Geometry: see drawing. Coordinates: mm, zero at the bounding-box minimum. Round coordinates to 2 decimals unless told otherwise and drop trailing zeros. Loops run counter-clockwise (first coordinate to the right, second up) from the corner with the lowest first, then second, coordinate; pieces in that order, holes last. Notation, with made-up numbers: (2.5, 28) - (57.5, 28) arc R22 ccw to (57.5, 49) - close; hole circle Ø7 at (-22, 88). An arc over 180 degrees is marked (long way). Return JSON: item names as keys, results as strings. Group by question number.
1. Material intervals for probe 1 along Y at (x, z) = (35, 3.45); probe 2 along Y at (x, z) = (35, 0.8); probe 3 along Z at (x, y) = (34, 43), sorted ascending.
2. First-contact query: pin 1 Ø3.5 at (x, y) = (35, 41.5) entering from +Z; pin 2 Ø3 at (y, z) = (30, 4) entering from +X; pin 3 Ø3 at (y, z) = (9, 1.5) entering from -X (3 decimals). Flat tips, straight axial feed; report the tip coordinate or a pass-through.
3. Section B-B on y = 35. Return loops of the section in (x, z), and give its area (3 significant figures).
4. Section C-C on z = 4.9. Return loops of the section in (x, y), and give its area (3 significant figures).
5. Section A-A on x = 35. Return loops of the section in (y, z).
6. Section D-D on y = 55. Return loops of the section in (x, z), and give its area (3 significant figures).
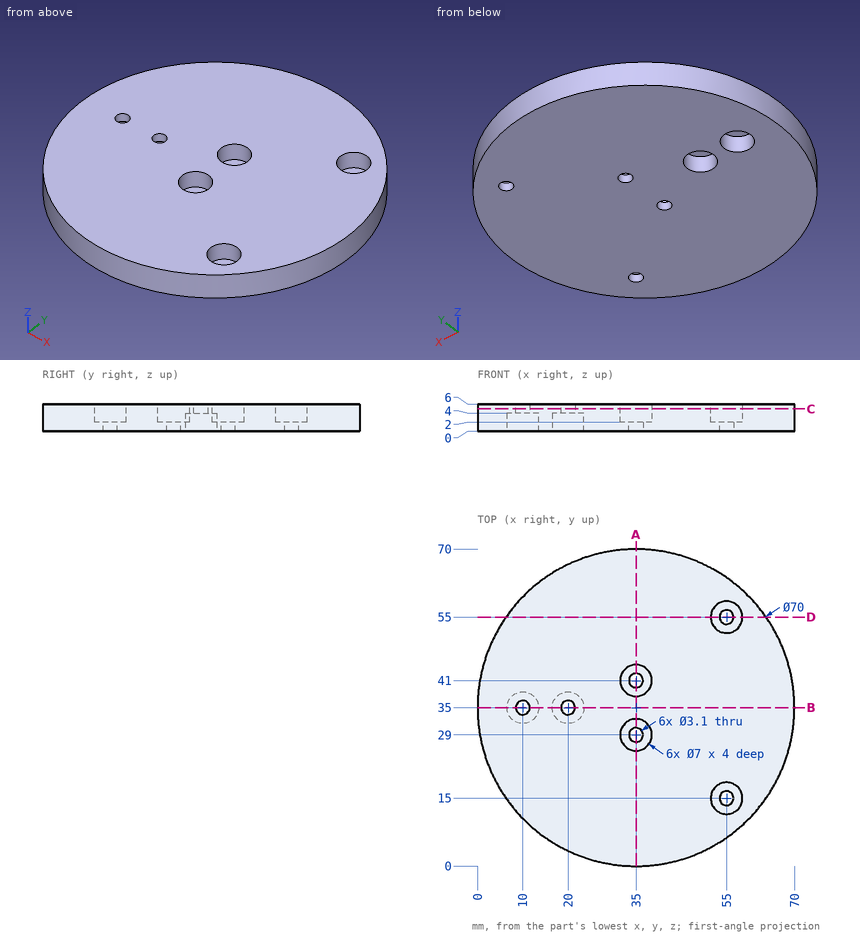
Taken from the geometry:
{
 "1": {"probe 1": "0 to 25.5, 32.5 to 37.5, 44.5 to 70", "probe 2": "0 to 27.45, 30.55 to 39.45, 42.55 to 70", "probe 3": "0 to 2"},
 "2": {"pin 1": "z = 2", "pin 2": "x = 69.82", "pin 3": "x = 10.005"},
 "3": {"outline": "(0, 0) - (6.5, 0) - (6.5, 4) - (8.45, 4) - (8.45, 6) - (0, 6) - close; (11.55, 4) - (13.5, 4) - (13.5, 0) - (16.5, 0) - (16.5, 4) - (18.45, 4) - (18.45, 6) - (11.55, 6) - close; (21.55, 4) - (23.5, 4) - (23.5, 0) - (70, 0) - (70, 6) - (21.55, 6) - close", "area": "352 mm2"},
 "4": {"outline": "circle Ø70 at (35, 35); hole circle Ø3.1 at (10, 35); hole circle Ø3.1 at (20, 35); hole circle Ø7 at (35, 29); hole circle Ø7 at (35, 41); hole circle Ø7 at (55, 15); hole circle Ø7 at (55, 55)", "area": "3,680 mm2"},
 "5": {"outline": "(0, 0) - (27.45, 0) - (27.45, 2) - (25.5, 2) - (25.5, 6) - (0, 6) - close; (30.55, 0) - (39.45, 0) - (39.45, 2) - (37.5, 2) - (37.5, 6) - (32.5, 6) - (32.5, 2) - (30.55, 2) - close; (42.55, 0) - (70, 0) - (70, 6) - (44.5, 6) - (44.5, 2) - (42.55, 2) - close"},
 "6": {"outline": "(6.28, 0) - (53.45, 0) - (53.45, 2) - (51.5, 2) - (51.5, 6) - (6.28, 6) - close; (56.55, 0) - (63.72, 0) - (63.72, 6) - (58.5, 6) - (58.5, 2) - (56.55, 2) - close", "area": "310 mm2"}
}
